```python
from build123d import *

# Parameters (mm, degrees)
F0_W     = 250
F0_H     = 210
F0_R     = 3.55
F1_DEPTH = 0.2


with BuildPart() as f1:
    # F0 (on Top) → F1 (new body)
    with BuildSketch(Plane.XY):
        Rectangle(F0_W, F0_H)
        with BuildLine():
            Line((-90.225, -104.55), (-124.55, -104.55))
            Line((-124.55, -104.55), (-124.55, -98.225))
            Line((-124.55, -98.225), (-93.993667, -98.225))
            ThreePointArc((-93.993667, -98.225), (-92.828427, -100.828427), (-90.225, -101.993667))
            Line((-90.225, -101.993667), (-90.225, -104.55))
        make_face(mode=Mode.SUBTRACT)
        with Locations((-90, -98)):
            Circle(F0_R, mode=Mode.SUBTRACT)
        with BuildLine():
            Line((-86.006333, -98.225), (8.006333, -98.225))
            ThreePointArc((8.006333, -98.225), (9.171573, -100.828427), (11.775, -101.993667))
            Line((11.775, -101.993667), (11.775, -104.55))
            Line((11.775, -104.55), (-89.775, -104.55))
            Line((-89.775, -104.55), (-89.775, -101.993667))
            ThreePointArc((-89.775, -101.993667), (-87.171573, -100.828427), (-86.006333, -98.225))
        make_face(mode=Mode.SUBTRACT)
        with BuildLine():
            Line((-124.55, -0.225), (-93.993667, -0.225))
            ThreePointArc((-93.993667, -0.225), (-92.828427, -2.828427), (-90.225, -3.993667))
            Line((-90.225, -3.993667), (-90.225, -94.006333))
            ThreePointArc((-90.225, -94.006333), (-92.828427, -95.171573), (-93.993667, -97.775))
            Line((-93.993667, -97.775), (-124.55, -97.775))
            Line((-124.55, -97.775), (-124.55, -0.225))
        make_face(mode=Mode.SUBTRACT)
        with BuildLine():
            Line((-86.006333, -0.225), (8.006333, -0.225))
            ThreePointArc((8.006333, -0.225), (9.171573, -2.828427), (11.775, -3.993667))
            Line((11.775, -3.993667), (11.775, -94.006333))
            ThreePointArc((11.775, -94.006333), (9.171573, -95.171573), (8.006333, -97.775))
            Line((8.006333, -97.775), (-86.006333, -97.775))
            ThreePointArc((-86.006333, -97.775), (-87.171573, -95.171573), (-89.775, -94.006333))
            Line((-89.775, -94.006333), (-89.775, -3.993667))
            ThreePointArc((-89.775, -3.993667), (-87.171573, -2.828427), (-86.006333, -0.225))
        make_face(mode=Mode.SUBTRACT)
        with Locations((12, -98)):
            Circle(F0_R, mode=Mode.SUBTRACT)
        with BuildLine():
            Line((12.225, -104.55), (12.225, -101.993667))
            ThreePointArc((12.225, -101.993667), (14.828427, -100.828427), (15.993667, -98.225))
            Line((15.993667, -98.225), (109.006333, -98.225))
            ThreePointArc((109.006333, -98.225), (110.171573, -100.828427), (112.775, -101.993667))
            Line((112.775, -101.993667), (112.775, -104.55))
            Line((112.775, -104.55), (12.225, -104.55))
        make_face(mode=Mode.SUBTRACT)
        with BuildLine():
            Line((124.55, -98.225), (124.55, -104.55))
            Line((124.55, -104.55), (113.225, -104.55))
            Line((113.225, -104.55), (113.225, -101.993667))
            ThreePointArc((113.225, -101.993667), (115.828427, -100.828427), (116.993667, -98.225))
            Line((116.993667, -98.225), (124.55, -98.225))
        make_face(mode=Mode.SUBTRACT)
        with Locations((113, -98)):
            Circle(F0_R, mode=Mode.SUBTRACT)
        with BuildLine():
            Line((15.993667, -0.225), (109.006333, -0.225))
            ThreePointArc((109.006333, -0.225), (110.171573, -2.828427), (112.775, -3.993667))
            Line((112.775, -3.993667), (112.775, -94.006333))
            ThreePointArc((112.775, -94.006333), (110.171573, -95.171573), (109.006333, -97.775))
            Line((109.006333, -97.775), (15.993667, -97.775))
            ThreePointArc((15.993667, -97.775), (14.828427, -95.171573), (12.225, -94.006333))
            Line((12.225, -94.006333), (12.225, -3.993667))
            ThreePointArc((12.225, -3.993667), (14.828427, -2.828427), (15.993667, -0.225))
        make_face(mode=Mode.SUBTRACT)
        with BuildLine():
            Line((116.993667, -0.225), (124.55, -0.225))
            Line((124.55, -0.225), (124.55, -97.775))
            Line((124.55, -97.775), (116.993667, -97.775))
            ThreePointArc((116.993667, -97.775), (115.828427, -95.171573), (113.225, -94.006333))
            Line((113.225, -94.006333), (113.225, -3.993667))
            ThreePointArc((113.225, -3.993667), (115.828427, -2.828427), (116.993667, -0.225))
        make_face(mode=Mode.SUBTRACT)
        with Locations((-90, 0)):
            Circle(F0_R, mode=Mode.SUBTRACT)
        with BuildLine():
            Line((-124.55, 97.775), (-93.993667, 97.775))
            ThreePointArc((-93.993667, 97.775), (-92.828427, 95.171573), (-90.225, 94.006333))
            Line((-90.225, 94.006333), (-90.225, 3.993667))
            ThreePointArc((-90.225, 3.993667), (-92.828427, 2.828427), (-93.993667, 0.225))
            Line((-93.993667, 0.225), (-124.55, 0.225))
            Line((-124.55, 0.225), (-124.55, 97.775))
        make_face(mode=Mode.SUBTRACT)
        with BuildLine():
            Line((-86.006333, 97.775), (8.006333, 97.775))
            ThreePointArc((8.006333, 97.775), (9.171573, 95.171573), (11.775, 94.006333))
            Line((11.775, 94.006333), (11.775, 3.993667))
            ThreePointArc((11.775, 3.993667), (9.171573, 2.828427), (8.006333, 0.225))
            Line((8.006333, 0.225), (-86.006333, 0.225))
            ThreePointArc((-86.006333, 0.225), (-87.171573, 2.828427), (-89.775, 3.993667))
            Line((-89.775, 3.993667), (-89.775, 94.006333))
            ThreePointArc((-89.775, 94.006333), (-87.171573, 95.171573), (-86.006333, 97.775))
        make_face(mode=Mode.SUBTRACT)
        with BuildLine():
            Line((-90.225, 104.55), (-90.225, 101.993667))
            ThreePointArc((-90.225, 101.993667), (-92.828427, 100.828427), (-93.993667, 98.225))
            Line((-93.993667, 98.225), (-124.55, 98.225))
            Line((-124.55, 98.225), (-124.55, 104.55))
            Line((-124.55, 104.55), (-90.225, 104.55))
        make_face(mode=Mode.SUBTRACT)
        with Locations((-90, 98)):
            Circle(F0_R, mode=Mode.SUBTRACT)
        with BuildLine():
            Line((-89.775, 101.993667), (-89.775, 104.55))
            Line((-89.775, 104.55), (11.775, 104.55))
            Line((11.775, 104.55), (11.775, 101.993667))
            ThreePointArc((11.775, 101.993667), (9.171573, 100.828427), (8.006333, 98.225))
            Line((8.006333, 98.225), (-86.006333, 98.225))
            ThreePointArc((-86.006333, 98.225), (-87.171573, 100.828427), (-89.775, 101.993667))
        make_face(mode=Mode.SUBTRACT)
        with Locations((12, 0)):
            Circle(F0_R, mode=Mode.SUBTRACT)
        with Locations((113, 0)):
            Circle(F0_R, mode=Mode.SUBTRACT)
        with BuildLine():
            Line((15.993667, 97.775), (109.006333, 97.775))
            ThreePointArc((109.006333, 97.775), (110.171573, 95.171573), (112.775, 94.006333))
            Line((112.775, 94.006333), (112.775, 3.993667))
            ThreePointArc((112.775, 3.993667), (110.171573, 2.828427), (109.006333, 0.225))
            Line((109.006333, 0.225), (15.993667, 0.225))
            ThreePointArc((15.993667, 0.225), (14.828427, 2.828427), (12.225, 3.993667))
            Line((12.225, 3.993667), (12.225, 94.006333))
            ThreePointArc((12.225, 94.006333), (14.828427, 95.171573), (15.993667, 97.775))
        make_face(mode=Mode.SUBTRACT)
        with BuildLine():
            Line((116.993667, 97.775), (124.55, 97.775))
            Line((124.55, 97.775), (124.55, 0.225))
            Line((124.55, 0.225), (116.993667, 0.225))
            ThreePointArc((116.993667, 0.225), (115.828427, 2.828427), (113.225, 3.993667))
            Line((113.225, 3.993667), (113.225, 94.006333))
            ThreePointArc((113.225, 94.006333), (115.828427, 95.171573), (116.993667, 97.775))
        make_face(mode=Mode.SUBTRACT)
        with Locations((12, 98)):
            Circle(F0_R, mode=Mode.SUBTRACT)
        with BuildLine():
            Line((12.225, 101.993667), (12.225, 104.55))
            Line((12.225, 104.55), (112.775, 104.55))
            Line((112.775, 104.55), (112.775, 101.993667))
            ThreePointArc((112.775, 101.993667), (110.171573, 100.828427), (109.006333, 98.225))
            Line((109.006333, 98.225), (15.993667, 98.225))
            ThreePointArc((15.993667, 98.225), (14.828427, 100.828427), (12.225, 101.993667))
        make_face(mode=Mode.SUBTRACT)
        with Locations((113, 98)):
            Circle(F0_R, mode=Mode.SUBTRACT)
        with BuildLine():
            Line((113.225, 104.55), (124.55, 104.55))
            Line((124.55, 104.55), (124.55, 98.225))
            Line((124.55, 98.225), (116.993667, 98.225))
            ThreePointArc((116.993667, 98.225), (115.828427, 100.828427), (113.225, 101.993667))
            Line((113.225, 101.993667), (113.225, 104.55))
        make_face(mode=Mode.SUBTRACT)
    extrude(amount=F1_DEPTH)


solid = f1.part
```
Design review of the part built by this model. Coordinates are the model's own, in mm. Coordinates: 2 decimals unless noted, no trailing zeros. Write each loop counter-clockwise with the first axis right and the second up, starting at its lowest first coordinate (ties: lowest second). Pieces come first, ordered by that corner, then holes.
1) Add section C-C (z = 0.15). State how many separate pieces and enclosed holes the cut face has, plus the area to 3 significant figures.
2) Add section B-B (x = -57). Write out the cut boundary in (y, z) (3 decimals).
3) To check wall thickness, follow L1, parallel to Y at x = -37, z = 0.1 (3 decimals); L2, parallel to Y at x = 113, z = 0.15; L3, parallel to X at y = 39, z = 0.1 (3 decimals). State the ranges of each line that lie inside material, in increasing order.
4) Add section A-A (y = -11.5). Write out the cut boundary in (x, z) (3 decimals), plus the area to 3 significant figures.
Check result:
1. separate pieces: 1
1. enclosed holes: 25
1. area: 1,060 mm2
2. outline: (-105, 0) - (-104.55, 0) - (-104.55, 0.2) - (-105, 0.2) - close; (-98.225, 0) - (-97.775, 0) - (-97.775, 0.2) - (-98.225, 0.2) - close; (-0.225, 0) - (0.225, 0) - (0.225, 0.2) - (-0.225, 0.2) - close; (97.775, 0) - (98.225, 0) - (98.225, 0.2) - (97.775, 0.2) - close; (104.55, 0) - (105, 0) - (105, 0.2) - (104.55, 0.2) - close
3. L1: y = -105 to -104.55, -98.225 to -97.775, -0.225 to 0.225, 97.775 to 98.225, 104.55 to 105
3. L2: y = -105 to -101.55, -94.45 to -3.55, 3.55 to 94.45, 101.55 to 105
3. L3: x = -125 to -124.55, -90.225 to -89.775, 11.775 to 12.225, 112.775 to 113.225, 124.55 to 125
4. outline: (-125, 0) - (-124.55, 0) - (-124.55, 0.2) - (-125, 0.2) - close; (-90.225, 0) - (-89.775, 0) - (-89.775, 0.2) - (-90.225, 0.2) - close; (11.775, 0) - (12.225, 0) - (12.225, 0.2) - (11.775, 0.2) - close; (112.775, 0) - (113.225, 0) - (113.225, 0.2) - (112.775, 0.2) - close; (124.55, 0) - (125, 0) - (125, 0.2) - (124.55, 0.2) - close
4. area: 0.450 mm2
